Source: three-view drawing plus pictorial views. Frame: mm from the lowest corner of the part. Give positions to 0.01 mm unless a question says otherwise; leave off trailing zeros. Order: outer loops, then holes, each group sorted by start corner. A loop starts at its lowest first (then second) coordinate and runs counter-clockwise, first axis right, second up. Notation, with made-up numbers: (21.25, -13) -> (29.25, -13) arc R29 ccw to (29.25, 22) -> close; hole circle Ø9 at (43, 55). An arc over 180 degrees is marked (long way). Answer in a Markdown table with one row per item. Add a question column.
Q1. Cut plane C-C on y = 9. Return the cut outline in (x, z).
Q2. Cut plane B-B on z = 10.25. Return the cut outline in (x, y), and give its area (3 significant figures).
Q3. Contact query for flat-ended pins moving along their axis: P1, Ø12, axis at x = 92, y = 5.5, coming from the -Z side; P2, Ø1.8, axis at x = 150, y = 12.5, coming from the +Z side. Output: stop coordinate, or through.
Q4. Cut plane A-A on x = 171.5. Return the cut outline in (y, z), and give its area (3 significant figures).
Q5. Line query: line 1 along Y through (x, z) = (50, 1.6); line 2 along Z through (x, y) = (118.5, 15); line 3 along X through (y, z) = (12, 2). Output: solid intervals per line, ascending. Write a range as from..to.
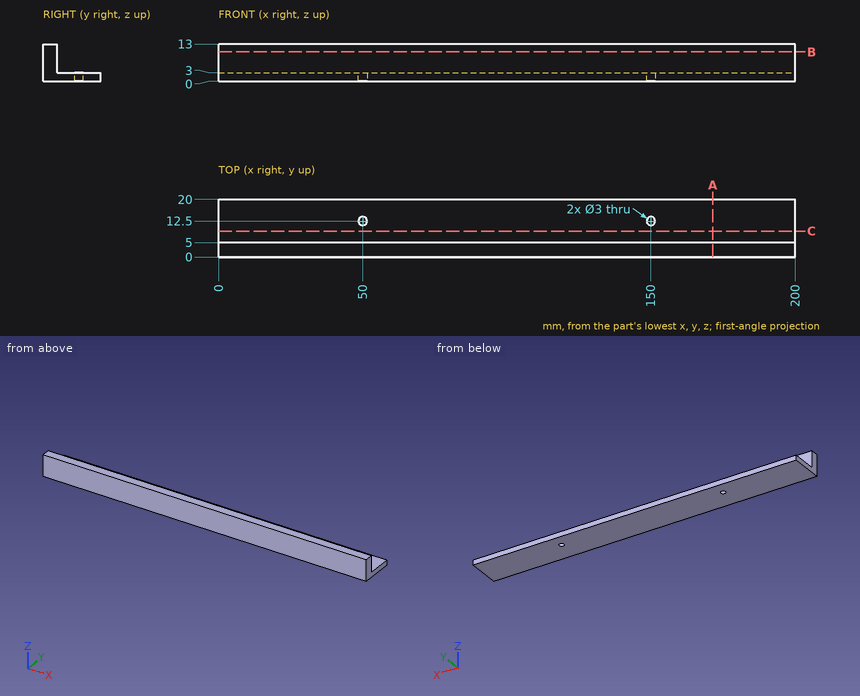
Completed:
| question | item | result |
|---|---|---|
| 1 | outline | (0, 0) -> (200, 0) -> (200, 3) -> (0, 3) -> close |
| 2 | outline | (0, 0) -> (200, 0) -> (200, 5) -> (0, 5) -> close |
| 2 | area | 1,000 mm² |
| 3 | P1 | stops at z = 0 |
| 3 | P2 | passes through |
| 4 | outline | (0, 0) -> (20, 0) -> (20, 3) -> (5, 3) -> (5, 13) -> (0, 13) -> close |
| 4 | area | 110 mm² |
| 5 | line 1 | y = 0..11, 14..20 |
| 5 | line 2 | z = 0..3 |
| 5 | line 3 | x = 0..48.59, 51.41..148.59, 151.41..200 |
